```python
from build123d import *

# Parameters (mm, degrees)
BOSS_EXTRUDE1_DEPTH = 5
SKETCH2_R           = 5.25
CUT_EXTRUDE1_DEPTH  = 25.779023387
SKETCH3_R           = 1.6
CUT_EXTRUDE2_DEPTH  = 22.118712082
FILLET1_R           = 2
FILLET2_R           = 1.5


with BuildPart() as part:
    # Sketch1 → Boss-Extrude1 (new, symmetric)
    with BuildSketch(Plane.XY):
        Polygon((-15, 0), (15, 0), (15, 3), (7, 3), (7, 17), (-7, 17), (-7, 3), (-15, 3), align=None)
    extrude(amount=BOSS_EXTRUDE1_DEPTH, both=True)

    # Sketch2 → Cut-Extrude1 (cut, through all)
    with BuildSketch(Plane.XY.offset(5)):
        with Locations((0, 10)):
            Circle(SKETCH2_R)
    extrude(amount=-CUT_EXTRUDE1_DEPTH, mode=Mode.SUBTRACT)

    # Sketch3 → Cut-Extrude2 (cut, through all)
    with BuildSketch(Plane(origin=(0, 3, 0), x_dir=(1, 0, 0), z_dir=(0, 1, 0))):
        with Locations(Location((11, 0, 0), (0, 0, 180))):
            Circle(SKETCH3_R)
        with Locations(Location((-11, 0, 0), (0, 0, 180))):
            Circle(SKETCH3_R)
    extrude(amount=-CUT_EXTRUDE2_DEPTH, mode=Mode.SUBTRACT)

    # Fillet1
    fillet1_edges = [part.edges().sort_by_distance(p)[0] for p in [
        (-7, 3, 0),
        (-7, 17, 0),
        (7, 17, 0),
        (7, 3, 0),
    ]]
    fillet(fillet1_edges, radius=FILLET1_R)

    # Fillet2
    fillet2_edges = [part.edges().sort_by_distance(p)[0] for p in [
        (-15, 0, 0),
        (-15, 3, 0),
        (15, 3, 0),
        (15, 0, 0),
    ]]
    fillet(fillet2_edges, radius=FILLET2_R - 0.0001)  # a hair under: the kernel refuses the full size


solid = part.part
```
Verification items for the finished model (mm, model axes). A direction names the side the tool comes from. Give positions to 0.01 mm unless a question says otherwise; leave off trailing zeros. Order: outer loops, then holes, each group sorted by start corner. A loop starts at its lowest first (then second) coordinate and runs counter-clockwise, first axis right, second up. Notation, with made-up numbers: (-37, 57.25) -> (22, 57.25) arc R28 cw to (22, 83.25) -> close; hole circle Ø6 at (69, 20.5). An arc over 180 degrees is marked (long way). Use a Markdown table: item, result.
1) Section check C-C, the plane y = 10. Record the boundary of the cut face in (x, z).
Results:
| item | result |
|---|---|
| outline | (-7, -5) -> (-5.25, -5) -> (-5.25, 5) -> (-7, 5) -> close; (5.25, -5) -> (7, -5) -> (7, 5) -> (5.25, 5) -> close |
2) Section check B-B, the plane x = 0. Record the boundary of the cut face in (y, z), then the cut area to 3 significant figures.
Results:
| item | result |
|---|---|
| outline | (0, -5) -> (4.75, -5) -> (4.75, 5) -> (0, 5) -> close; (15.25, -5) -> (17, -5) -> (17, 5) -> (15.25, 5) -> close |
| area | 65.0 mm² |
3) Depth check by flat-ended pin: pin 1 Ø3 at (x, z) = (-11, 0) entering from +Y; pin 2 Ø2.5 at (x, z) = (11, 1.5) entering from +Y; pin 3 Ø2 at (y, z) = (10, -3) entering from +X; pin 4 Ø2 at (y, z) = (3, 3.5) entering from +X. Enter the tip coordinate at first touch or a pass-through.
Results:
| item | result |
|---|---|
| pin 1 | through |
| pin 2 | y = 3 |
| pin 3 | x = 7 |
| pin 4 | x = 14.91 |
4) Mould release check, pull along Z, two halves, no side actions. Record for faces 4 (the flat face through (3, 5, -5)), 5 (the cylindrical face through (-14.57, 0.45, -0.07)), 6 (the cylindrical face through (12.6, 1.52, 0.07)): pulls with the +Z half, pulls with the -Z half, needs draft (parallel to the pull), parting line crosses it, or undercut.
Results:
| item | result |
|---|---|
| face 4 | pulls with the -Z half |
| face 5 | needs draft |
| face 6 | undercut |
5) Tool access check on faces 1 (the flat face through (-7, 10, 0)), 2 (the cylindrical face through (14.55, 0.43, 0.07)), 3 (the flat face through (13, 3, 0)). Record the directions out of +Z, -Z, +X, -X, +Y, -Y that give a thin tool (end or side, any length) a straight path to the whole face; none if there is none.
Results:
| item | result |
|---|---|
| face 1 | +Z, -Z, -X, +Y |
| face 2 | +Z, -Z, +X, -Y |
| face 3 | +Z, -Z, +X, +Y |
6) Material ranges on probe 1 along Z at (x, y) = (11, 1.4); probe 2 along Y at (x, z) = (-13.25, 4.25); probe 3 along X at (y, z) = (12.5, -4.25), recorded low to high.
Results:
| item | result |
|---|---|
| probe 1 | -5 to -1.6, 1.6 to 5 |
| probe 2 | 0 to 3 |
| probe 3 | -7 to -4.62, 4.62 to 7 |
7) Section check A-A, the plane z = 0. Give the number of separate pieces and of enclosed holes in the cut face, then the cut area to 3 significant figures.
Results:
| item | result |
|---|---|
| separate pieces | 3 |
| enclosed holes | 1 |
| area | 178 mm² |
